Check sheet for the modelled part. Datum: model origin and axes. Units: mm. Face numbers are marked on the shaded views. Coordinates: 2 decimals unless noted, no trailing zeros. Loops run counter-clockwise (first coordinate to the right, second up) from the corner with the lowest first, then second, coordinate; pieces in that order, holes last. Notation, with made-up numbers: M 5.25,-16.75 L 37.25,-16.75 A18 cw 37.25,-12.75 Z; hole C -8,1 d4. An arc over 180 degrees is marked long. Return JSON: item names as keys, results as strings.
from build123d import *

# Parameters (mm, degrees)
SKETCH_R        = 42
PAD_DEPTH       = 2
SKETCH001_R     = 27.5
SKETCH001_R_2   = 20
PAD001_DEPTH    = 5
SKETCH002_R     = 22.5
SKETCH002_R_2   = 20
PAD002_DEPTH    = 10
CHAMFER_SIZE    = 1
SKETCH003_R     = 2
POCKET_DEPTH    = 2.001
SKETCH004_R     = 10
POCKET001_DEPTH = 5
SKETCH005_R     = 4.5
POCKET002_DEPTH = 2.001


with BuildPart() as part:
    # Sketch → Pad (new body)
    with BuildSketch(Plane.XY):
        Circle(SKETCH_R)
    extrude(amount=PAD_DEPTH)

    # Sketch001 (on Face3 of Pad) → Pad001 (join)
    with BuildSketch(Plane.XY.offset(2)):
        Circle(SKETCH001_R)
        Circle(SKETCH001_R_2, mode=Mode.SUBTRACT)
    extrude(amount=PAD001_DEPTH)

    # Sketch002 (on Face5 of Pad001) → Pad002 (join)
    with BuildSketch(Plane.XY.offset(7)):
        Circle(SKETCH002_R)
        Circle(SKETCH002_R_2, mode=Mode.SUBTRACT)
    extrude(amount=PAD002_DEPTH)

    # Chamfer
    chamfer_edges = [part.edges().sort_by_distance(p)[0] for p in [
        (-22.5, 0, 17),
    ]]
    chamfer(chamfer_edges, length=CHAMFER_SIZE)

    # Sketch003 (on Face10 of Chamfer) → Pocket (cut, through all)
    with BuildSketch(Plane.XY.offset(2)):
        with Locations((-10, 10)):
            Circle(SKETCH003_R)
        with Locations((10, 10)):
            Circle(SKETCH003_R)
        with Locations((10, -10)):
            Circle(SKETCH003_R)
        with Locations((-10, -10)):
            Circle(SKETCH003_R)
    extrude(amount=-POCKET_DEPTH, mode=Mode.SUBTRACT)

    # Sketch004 (on Face10 of Pocket) → Pocket001 (cut)
    with BuildSketch(Plane.XY.offset(2)):
        Circle(SKETCH004_R)
    extrude(amount=-POCKET001_DEPTH, mode=Mode.SUBTRACT)

    # Sketch005 (on Face7 of Pocket001) → Pocket002 (cut, through all)
    with BuildSketch(Plane.XY.offset(2)):
        with Locations((-22.98097, 22.98097)):
            Circle(SKETCH005_R)
        with Locations((0, 32.5)):
            Circle(SKETCH005_R)
        with Locations((22.98097, 22.98097)):
            Circle(SKETCH005_R)
        with Locations((32.5, 0)):
            Circle(SKETCH005_R)
        with Locations((-32.5, 0)):
            Circle(SKETCH005_R)
        with Locations((-22.98097, -22.98097)):
            Circle(SKETCH005_R)
        with Locations((0, -32.5)):
            Circle(SKETCH005_R)
        with Locations((22.98097, -22.98097)):
            Circle(SKETCH005_R)
    extrude(amount=-POCKET002_DEPTH, mode=Mode.SUBTRACT)


solid = part.part
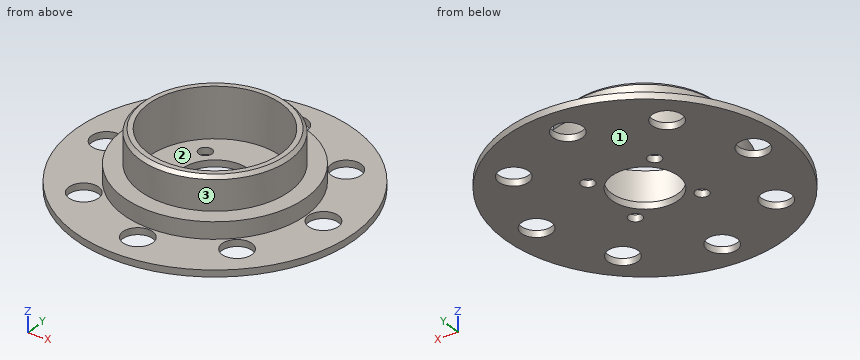
1) Section check A-A on x = 0. Count the separate pieces of the cut face and the enclosed holes in it, then the cut area to 3 significant figures.
Answers:
{"separate pieces": "4", "enclosed holes": "0", "area": "216 mm²"}
2) Scan lines: line 1 along Y through (x, z) = (0, 0.7); line 2 along Z through (x, y) = (24.5, 4); line 3 along Z through (x, y) = (-34.5, -15). Record each from-to range of solid material in increasing order. Write a range as [from, to].
Answers:
{"line 1": "[-42, -37], [-28, -10], [10, 28], [37, 42]", "line 2": "[0, 7]", "line 3": "[0, 2]"}
3) Section check C-C on y = -26.5. Record the cut outline in (x, z), then the cut area to 3 significant figures.
Answers:
{"outline": "M -32.58,0 L -25.79,0 L -25.79,2 L -32.58,2 Z; M -20.18,0 L 20.18,0 L 20.18,2 L 7.35,2 L 7.35,7 L -7.35,7 L -7.35,2 L -20.18,2 Z; M 25.79,0 L 32.58,0 L 32.58,2 L 25.79,2 Z", "area": "181 mm²"}
4) Section check D-D on z = 3. Record the cut outline in (x, y).
Answers:
{"outline": "C 0,0 d55; hole C 0,0 d40"}
5) Go/stop test with flat-tipped pins: pin 1 Ø2 at (y, z) = (-10, 5) entering from -X; pin 2 Ø2 at (x, y) = (33.5, -3.5) entering from +Z; pin 3 Ø10 at (y, z) = (7, 11) entering from -X. Record where each tip stops, or that it passes through.
Answers:
{"pin 1": "x = -25.99", "pin 2": "z = 2", "pin 3": "x = -27.21"}
6) Draft check along Y on the marked faces 1, 2 and 3. Enter one of: +Y half, -Y half, draft (parallel to the pull), parting line (faces both ways), or undercut.
Answers:
{"face 1": "draft", "face 2": "undercut", "face 3": "parting line"}
